Input: dimensioned drawing with shaded views. Units: mm. Origin: part minimum x, y, z. A direction names the side the tool comes from. Coordinates: 2 decimals unless noted, no trailing zeros. Loops run counter-clockwise (first coordinate to the right, second up) from the corner with the lowest first, then second, coordinate; pieces in that order, holes last. Notation, with made-up numbers: (85.25, 62) - (98.25, 62) arc R25 cw to (98.25, 94) - close; hole circle Ø1 at (-4.5, 18). An arc over 180 degrees is marked (long way). Put each result on its own line as item: value. Start each with the question number.
1) Material intervals for line 1 along Y through (x, z) = (93, 15); line 2 along X through (y, z) = (33.5, 88), sorted ascending. Write a range as from..to.
2) Section C-C on y = 55. Output: boundary loops of the cut face in (x, z).
3) Section A-A on z = 21. Output: boundary loops of the cut face in (x, y), and give its area (3 significant figures).
4) Reachability of the marked faces 1 and 2 from +Z, -Z, +X, -X, +Y, -Y: full face, straight path, thin tool, end or side. Return the list, or none.
5) Section B-B on x = 93. Output: boundary loops of the cut face in (y, z).
6) Contact query for flat-ended pins moving along their axis: pin 1 Ø11.5 at (y, z) = (56.5, 43) entering from +X; pin 2 Ø2 at (x, z) = (85.5, 21.5) entering from +Y; pin 3 Ø1.5 at (x, y) = (26, 57) entering from -Z. Output: stop coordinate, or through.
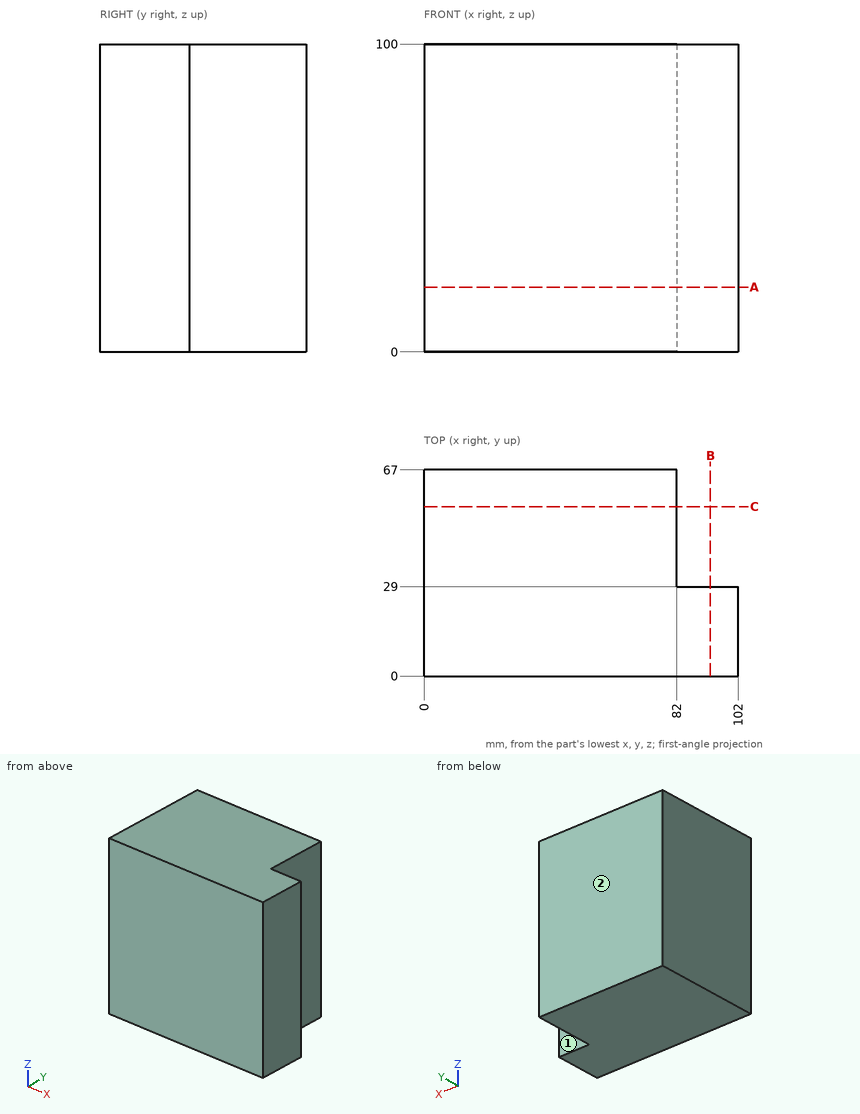
Answer block:
1. line 1: y = 0..29
1. line 2: x = 0..82
2. outline: (0, 0) - (82, 0) - (82, 100) - (0, 100) - close
3. outline: (0, 0) - (102, 0) - (102, 29) - (82, 29) - (82, 67) - (0, 67) - close
3. area: 6,070 mm²
4. face 1: +Z, -Z, +X, +Y
4. face 2: +Z, -Z, +X, -X, +Y
5. outline: (0, 0) - (29, 0) - (29, 100) - (0, 100) - close
6. pin 1: stops at x = 82
6. pin 2: stops at y = 29
6. pin 3: stops at z = 0
